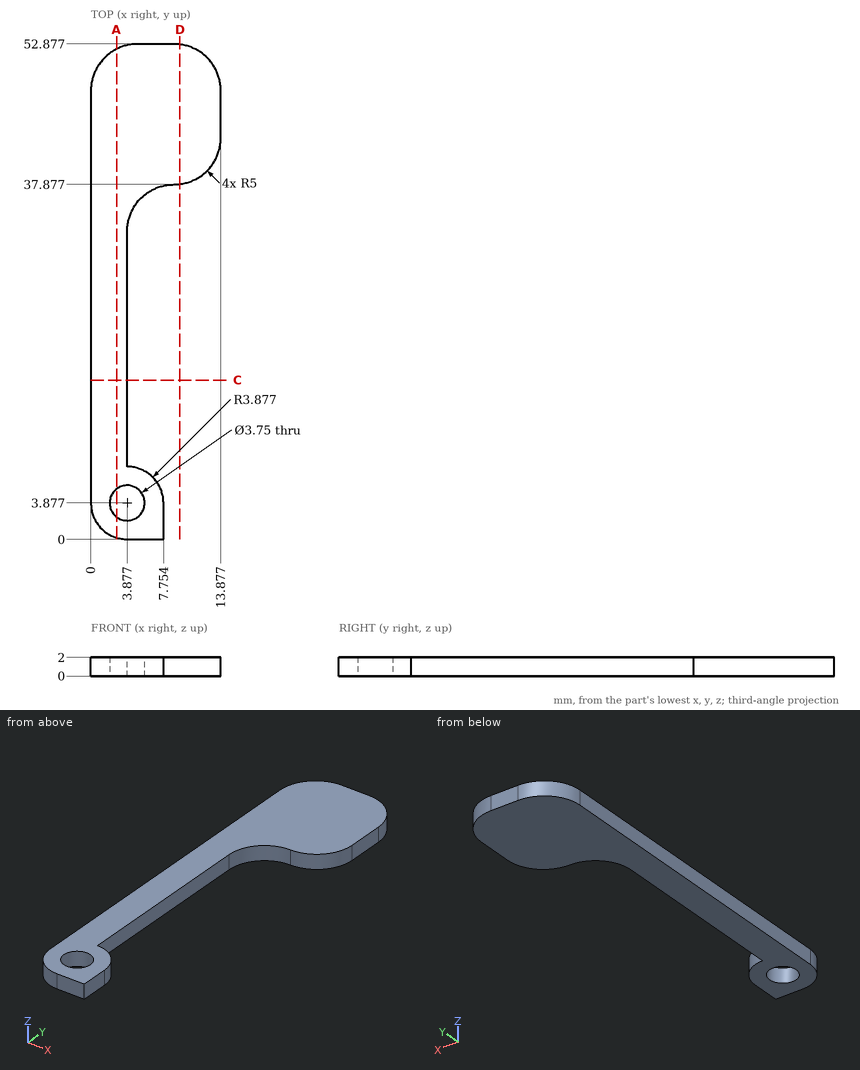
Geometry check sheet. Reference: drawing and pictorial views, mm from the part's lowest x, y, z. Round coordinates to 2 decimals unless told otherwise and drop trailing zeros. Order: outer loops, then holes, each group sorted by start corner. A loop starts at its lowest first (then second) coordinate and runs counter-clockwise, first axis right, second up.
Q1. Depth check by flat-ended pin: P1, Ø1.5, axis at x = 10.5, y = 45.5, coming from the -Z side; P2, Ø1, axis at x = 3, z = 0.5, coming from the +Y side. Enter the tip coordinate at first touch or a pass-through.
Filled sheet:
P1: stops at z = 0
P2: stops at y = 52.65
Q2. Cross-section at C-C, the plane y = 17. Enter the section's corners in (x, z).
Filled sheet:
outline: (0, 0) - (3.88, 0) - (3.88, 2) - (0, 2) - close
Q3. Cross-section at A-A, the plane x = 2.75. Enter the section's corners in (y, z).
Filled sheet:
outline: (0.17, 0) - (2.38, 0) - (2.38, 2) - (0.17, 2) - close; (5.38, 0) - (52.34, 0) - (52.34, 2) - (5.38, 2) - close
Q4. Cross-section at D-D, the plane x = 9.5. Enter the section's corners in (y, z).
Filled sheet:
outline: (37.92, 0) - (52.84, 0) - (52.84, 2) - (37.92, 2) - close
Q5. Scan lines: L1, parallel to Y at x = 5, z = 1.5 (1 decimal); L2, parallel to X at y = 27.5, z = 1.55; L3, parallel to Y at x = 2.75, z = 0.85 (1 decimal). Record each from-to range of solid material in increasing order.
Filled sheet:
L1: y = 0 to 2.4, 5.4 to 7.6, 36 to 52.9
L2: x = 0 to 3.88
L3: y = 0.2 to 2.4, 5.4 to 52.3
